Input: part model. Units: mm. Frame: model coordinates. A direction names the side the tool comes from. Round coordinates to 2 decimals unless told otherwise and drop trailing zeros. Loops run counter-clockwise (first coordinate to the right, second up) from the corner with the lowest first, then second, coordinate; pieces in that order, holes last.
(1) Cut plane B-B, the plane x = 67. Output: boundary loops of the cut face in (y, z), and give its area (3 significant figures).
(2) Cut plane A-A, the plane y = -102.25. Output: boundary loops of the cut face in (x, z).
(3) Line query: line 1 (X direction, y = -120.5, z = -57.5); line 2 (X direction, y = -114, z = -3); line 3 (Y direction, x = 105, z = -26.5). Output: solid intervals per line, ascending.
(4) First-contact query: pin 1 Ø3 at (x, z) = (103, -83.5) entering from +Y; pin 2 Ø12 at (x, z) = (86.5, -88.5) entering from +Y; pin 3 Ø2.5 at (x, z) = (108, -115) entering from +Y. Flat tips, straight axial feed; report the tip coordinate or a pass-through.
(5) Access query for faces 4 (the face through (113.616, -120.735, -141.955)), 5 (the face through (50, -105.2, -175)), 6 (the face through (31.733, -116.167, 37.535)). Directions: +Z, -Z, +X, -X, +Y, -Y. A direction counts if a zero-diameter tool reaches every point of the face in a straight line with its end or side. Return the directions, or none.
(6) Draft query along Y for faces 1 (the face through (99.95, -118.11, 37.53)), 2 (the face through (24, -101, -175)), 3 (the face through (113, -118.2, -140)). Return one class per face: released by +Y, released by -Y, zero draft, split by the parting line, or undercut.
from build123d import *
from build123d.topology import SkipClean

# Parameters (mm, degrees)
EXTRUDE_1_DEPTH     = 170
CHAMFER_1_SIZE      = 8
SKETCH_2_W          = 170
SKETCH_2_H          = 10
CUT_EXTRUDE_1_DEPTH = 0.84
EXTRUDE_2_DEPTH     = 80
SKETCH_4_W          = 250
SKETCH_4_H          = 10
CUT_EXTRUDE_2_DEPTH = 12
SKETCH_5_W          = 101.997424074
SKETCH_5_H          = 18
EXTRUDE_3_DEPTH     = 10
SKETCH_6_R          = 2.05
CUT_EXTRUDE_3_DEPTH = 5
SKETCH_7_W          = 16
SKETCH_7_H          = 10
EXTRUDE_4_DEPTH     = 8.2
CUT_EXTRUDE_5_DEPTH = 40
SKETCH_11_R         = 2.05
CUT_EXTRUDE_6_DEPTH = 5


with BuildPart() as part:
    # 草图1 → 凸台-拉伸1 (new body)
    with BuildSketch(Plane.XY):
        Polygon((28.8, -113.2), (35.2, -113.2), (35.2, -105.2), (40, -105.2), (40, -113.2), (59, -113.2), (59, -105.2), (63.8, -105.2), (63.8, -113.2), (70.2, -113.2), (70.2, -105.2), (75, -105.2), (75, -113.2), (94, -113.2), (94, -105.2), (98.8, -105.2), (98.8, -113.2), (105.2, -113.2), (105.2, -105.2), (110, -105.2), (110, -113.2), (130, -113.2), (130, -123.2), (15.162575926, -123.2), (15.162575926, -113.2), (24, -113.2), (24, -105.2), (28.8, -105.2), align=None)
    extrude(amount=-EXTRUDE_1_DEPTH)

    # 倒角1
    chamfer_1_edges = [part.edges().sort_by_distance(p)[0] for p in [
        (24, -113.2, -85),
        (110, -113.2, -85),
        (94, -113.2, -85),
        (75, -113.2, -85),
        (59, -113.2, -85),
        (40, -113.2, -85),
    ]]
    chamfer(chamfer_1_edges, length=CHAMFER_1_SIZE - 0.0001)  # a hair under: the kernel refuses the full size

    # 草图2 → 切除-拉伸1 (cut)
    with BuildSketch(Plane.ZY.offset(-15.162575926)):
        with Locations((-85, -118.2)):
            Rectangle(SKETCH_2_W, SKETCH_2_H)
    extrude(amount=-CUT_EXTRUDE_1_DEPTH, mode=Mode.SUBTRACT)

    # 草图3 → 凸台-拉伸2 (add)
    with SkipClean():  # the faces are left unmerged after this step: merging them gives an invalid solid
        with BuildSketch(Plane.XY):
            Polygon((24, -105.2), (16, -113.2), (16.002575926, -113.2), (16.002575926, -123.2), (130, -123.2), (130, -113.2), (118, -113.2), (110, -105.2), (105.2, -105.2), (105.2, -113.2), (98.8, -113.2), (98.8, -105.2), (94, -105.2), (86, -113.2), (83, -113.2), (75, -105.2), (70.2, -105.2), (70.2, -113.2), (63.8, -113.2), (63.8, -105.2), (59, -105.2), (51, -113.2), (48, -113.2), (40, -105.2), (35.2, -105.2), (35.2, -113.2), (28.8, -113.2), (28.8, -105.2), align=None)
        extrude(amount=EXTRUDE_2_DEPTH)

    # 草图4 → 切除-拉伸2 (cut)
    with SkipClean():  # the faces are left unmerged after this step: merging them gives an invalid solid
        with BuildSketch(Plane(origin=(130, 0, 0), x_dir=(0, 0, -1), z_dir=(1, 0, 0))):
            with Locations((45, -118.2)):
                Rectangle(SKETCH_4_W, SKETCH_4_H)
        extrude(amount=-CUT_EXTRUDE_2_DEPTH, mode=Mode.SUBTRACT)

    # 草图5 → 凸台-拉伸3 (add)
    with SkipClean():  # the faces are left unmerged after this step: merging them gives an invalid solid
        with BuildSketch(Plane(origin=(0, 0, -170), x_dir=(-1, 0, 0), z_dir=(0, 0, -1))):
            with Locations((-67.001287963, -114.2)):
                Rectangle(SKETCH_5_W, SKETCH_5_H)
        extrude(amount=EXTRUDE_3_DEPTH)

    # 草图6 → 切除-拉伸3 (cut)
    with SkipClean():  # the faces are left unmerged after this step: merging them gives an invalid solid
        with BuildSketch(Plane.XZ.offset(123.2)):
            with Locations(Location((21.002575926, 25, 0), (0, 0, 270))):
                Circle(SKETCH_6_R)
            with Locations(Location((21.002575926, 0, 0), (0, 0, 270))):
                Circle(SKETCH_6_R)
            with Locations(Location((21.002575926, -57.5, 0), (0, 0, 270))):
                Circle(SKETCH_6_R)
            with Locations(Location((21.002575926, -82.5, 0), (0, 0, 270))):
                Circle(SKETCH_6_R)
            with Locations(Location((21.002575926, -140, 0), (0, 0, 270))):
                Circle(SKETCH_6_R)
            with Locations(Location((21.002575926, -165, 0), (0, 0, 270))):
                Circle(SKETCH_6_R)
            with Locations(Location((113, -140, 0), (0, 0, 270))):
                Circle(SKETCH_6_R)
            with Locations(Location((113, -82.5, 0), (0, 0, 270))):
                Circle(SKETCH_6_R)
            with Locations(Location((113, -57.5, 0), (0, 0, 270))):
                Circle(SKETCH_6_R)
            with Locations(Location((113, 0, 0), (0, 0, 270))):
                Circle(SKETCH_6_R)
            with Locations(Location((113, 25, 0), (0, 0, 270))):
                Circle(SKETCH_6_R)
            with Locations(Location((113, -165, 0), (0, 0, 270))):
                Circle(SKETCH_6_R)
        extrude(amount=-CUT_EXTRUDE_3_DEPTH, mode=Mode.SUBTRACT)

    # 草图7 → 凸台-拉伸4 (add)
    with SkipClean():  # the faces are left unmerged after this step: merging them gives an invalid solid
        with BuildSketch(Plane(origin=(0, -105.2, 0), x_dir=(1, 0, 0), z_dir=(0, 1, 0))):
            with Locations((102, 175)):
                Rectangle(SKETCH_7_W, SKETCH_7_H)
            with Locations((67, 175)):
                Rectangle(SKETCH_7_W, SKETCH_7_H)
            with Locations((32, 175)):
                Rectangle(SKETCH_7_W, SKETCH_7_H)
        extrude(amount=EXTRUDE_4_DEPTH)

    # 草图10 → 切除-拉伸5 (cut)
    with SkipClean():  # the faces are left unmerged after this step: merging them gives an invalid solid
        with BuildSketch(Plane.XY.offset(80)):
            Polygon((16.002575926, -123.2), (118, -123.2), (118, -113.2), (110, -105.2), (105.2, -105.2), (105.2, -113.2), (98.8, -113.2), (98.8, -105.2), (94, -105.2), (86, -113.2), (83, -113.2), (75, -105.2), (70.2, -105.2), (70.2, -113.2), (63.8, -113.2), (63.8, -105.2), (59, -105.2), (51, -113.2), (48, -113.2), (40, -105.2), (35.2, -105.2), (35.2, -113.2), (28.8, -113.2), (28.8, -105.2), (24, -105.2), (16, -113.2), (16.002575926, -113.2), align=None)
        extrude(amount=-CUT_EXTRUDE_5_DEPTH, mode=Mode.SUBTRACT)

    # 草图11 → 切除-拉伸6 (cut)
    with SkipClean():  # the faces are left unmerged after this step: merging them gives an invalid solid
        with BuildSketch(Plane.XY.offset(40)):
            with Locations((32, -118.2)):
                Circle(SKETCH_11_R)
            with Locations((67, -118.2)):
                Circle(SKETCH_11_R)
            with Locations((102, -118.2)):
                Circle(SKETCH_11_R)
        extrude(amount=-CUT_EXTRUDE_6_DEPTH, mode=Mode.SUBTRACT)


solid = part.part
Reported:
1. outline: (-123.2, -180) - (-97, -180) - (-97, -170) - (-113.2, -170) - (-113.2, 40) - (-116.15, 40) - (-116.15, 35) - (-120.25, 35) - (-120.25, 40) - (-123.2, 40) - close
1. area: 2,340 mm2
2. outline: (24, -180) - (40, -180) - (40, -170) - (24, -170) - close; (59, -180) - (75, -180) - (75, -170) - (59, -170) - close; (94, -180) - (110, -180) - (110, -170) - (94, -170) - close
3. line 1: x = 16 to 18.95, 23.05 to 110.95, 115.05 to 118
3. line 2: x = 16 to 118
3. line 3: y = -123.2 to -113.2
4. pin 1: stops at y = -113.2
4. pin 2: stops at y = -106.7
4. pin 3: stops at y = -105.2
5. face 4: -Y
5. face 5: +Z, -Z, +Y
5. face 6: +Z
6. face 1: undercut
6. face 2: zero draft
6. face 3: released by -Y
